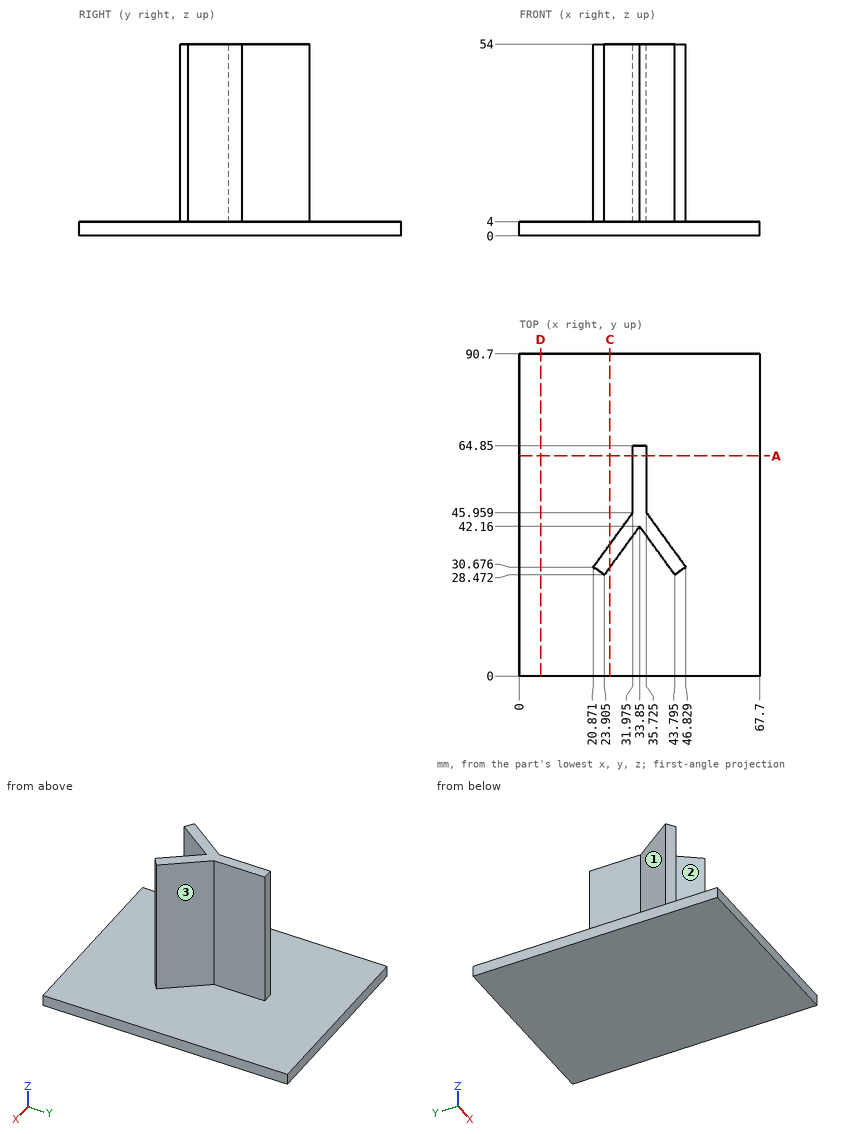
Check sheet for the drawn part. Datum: minimum x, y, z corner. Units: mm. A direction names the side the tool comes from. Give positions to 0.01 mm unless a question says otherwise; leave off trailing zeros. Order: outer loops, then holes, each group sorted by start corner. A loop starts at its lowest first (then second) coordinate and runs counter-clockwise, first axis right, second up. Notation, with made-up numbers: (-25, -19.5) - (29, -19.5) arc R21 ccw to (29, -7.5) - close; hole circle Ø7 at (-32.5, 19.5). An arc over 180 degrees is marked (long way). Write item = value, one per line. Start each with the question number.
1) Section check C-C (x = 25.5). Enter the section's corners in (y, z), then the cut area to 3 significant figures.
2) Section check D-D (x = 6). Enter the section's corners in (y, z), then the cut area to 3 significant figures.
3) Scan lines: L1, parallel to Z at x = 64.5, y = 48; L2, parallel to Y at x = 37.5, z = 24 (1 decimal); L3, parallel to X at y = 62.5, z = 12 (1 decimal). Record each from-to range of solid material in increasing order.
4) Section check A-A (y = 62). Enter the section's corners in (x, z) (1 decimal), then the cut area to 3 significant figures.
5) Access from +Z, -Z, +X, -X, +Y, -Y to the whole of each face (thin tool, end or side, straight path). Record for the marked faces 1, 2 and 3.
6) Gauge pin test, flat ends, axial feed: pin 1 Ø10 at (y, z) = (41.5, 43) entering from -X; pin 2 Ø10 at (x, y) = (48, 78) entering from +Z; pin 3 Ø2 at (x, z) = (36.5, 30.5) entering from +Y. Record the tip position at first contact, or that the pin passes through.
Geometry check:
q1.outline = (0, 0) - (90.7, 0) - (90.7, 4) - (37.05, 4) - (37.05, 54) - (30.67, 54) - (30.67, 4) - (0, 4) - close
q1.area = 682 mm2
q2.outline = (0, 0) - (90.7, 0) - (90.7, 4) - (0, 4) - close
q2.area = 363 mm2
q3.L1 = 0 to 4
q3.L2 = 37.1 to 43.5
q3.L3 = 32 to 35.7
q4.outline = (0, 0) - (67.7, 0) - (67.7, 4) - (35.7, 4) - (35.7, 54) - (32, 54) - (32, 4) - (0, 4) - close
q4.area = 458 mm2
q5.face_1 = +Z, -X, +Y
q5.face_2 = +Z, -Y
q5.face_3 = +Z, +X, +Y
q6.pin_1 = 25.1
q6.pin_2 = 4
q6.pin_3 = 64.85
